CAD build for the part. Positions are in the model's coordinates, mm. Round coordinates to 2 decimals unless told otherwise and drop trailing zeros. Write each loop counter-clockwise with the first axis right and the second up, starting at its lowest first coordinate (ties: lowest second). Pieces come first, ordered by that corner, then holes. Notation, with made-up numbers: (53, -8) - (83, -8) arc R20 ccw to (83, 27) - close; hole circle Ø9 at (34.25, -8). An arc over 180 degrees is marked (long way). Put each result on its own line as item: value. Start each with the question number.
Item 1: Drill centre lines: line 1 (Y direction, x = 0, z = 5.75); line 2 (X direction, y = -4, z = 5.5); line 3 (X direction, y = 54.5, z = 4.25). Where is each one in solid material? Low to high. Write a range as from..to.
Item 2: Cut at A-A (z = 15). Give the cut face in (x, y), and give its area (3 significant figures).
Item 3: Cut at B-B (y = 0). Give the cut face in (x, z), and give its area (3 significant figures).
Item 4: Cut at D-D (x = 16). Give the cut face in (y, z), and give its area (3 significant figures).
Item 5: Mould opens along X. For faces 1 (the flat face through (-25, -1, 10)), 2 (the cylindrical face through (0, 40, 10)), 3 (the flat face through (23, -60, 10)) say: released by +X, released by -X, zero draft, split by the parting line, or undercut.
Item 6: Cut at C-C (x = 1.5). Give the cut face in (y, z), and give its area (3 significant figures).
Item 7: Pin check, flat tips, straight feed: pin 1 Ø8 at (x, y) = (19.5, 13) entering from -Z; pin 2 Ø2 at (x, z) = (-11.5, 3.5) entering from -Y; pin 3 Ø6 at (x, z) = (5.5, 12) entering from -Y. Stop position of each tip, or through.
```python
from build123d import *

# Parameters (mm, degrees)
SKETCH1_R           = 5.25
BOSS_EXTRUDE1_DEPTH = 20


with BuildPart() as part:
    # Sketch1 → Boss-Extrude1 (new body)
    with BuildSketch(Plane.XY):
        with BuildLine():
            Line((20, 60), (25, 60))
            Line((25, 60), (25, -60))
            Line((25, -60), (20, -60))
            ThreePointArc((20, -60), (0, -40), (-20, -60))
            Line((-20, -60), (-25, -60))
            Line((-25, -60), (-25, 60))
            Line((-25, 60), (-20, 60))
            ThreePointArc((-20, 60), (0, 40), (20, 60))
        make_face()
        Circle(SKETCH1_R, mode=Mode.SUBTRACT)
    extrude(amount=BOSS_EXTRUDE1_DEPTH)


solid = part.part
```
Output values:
1. line 1: -40..-5.25, 5.25..40
1. line 2: -25..-3.4, 3.4..25
1. line 3: -25..-19.23, 19.23..25
2. outline: (-25, -60) - (-20, -60) arc R20 cw to (20, -60) - (25, -60) - (25, 60) - (20, 60) arc R20 cw to (-20, 60) - (-25, 60) - close; hole circle Ø10.5 at (0, 0)
2. area: 4,660 mm2
3. outline: (-25, 0) - (-5.25, 0) - (-5.25, 20) - (-25, 20) - close; (5.25, 0) - (25, 0) - (25, 20) - (5.25, 20) - close
3. area: 790 mm2
4. outline: (-48, 0) - (48, 0) - (48, 20) - (-48, 20) - close
4. area: 1,920 mm2
5. face 1: released by -X
5. face 2: undercut
5. face 3: zero draft
6. outline: (-40.06, 0) - (-5.03, 0) - (-5.03, 20) - (-40.06, 20) - close; (5.03, 0) - (40.06, 0) - (40.06, 20) - (5.03, 20) - close
6. area: 1,400 mm2
7. pin 1: z = 0
7. pin 2: y = -44.39
7. pin 3: y = -41.9
